Source: three-view drawing plus pictorial views. Frame: mm from the lowest corner of the part. A direction names the side the tool comes from. Round coordinates to 2 decimals unless told otherwise and drop trailing zeros. Loops run counter-clockwise (first coordinate to the right, second up) from the corner with the lowest first, then second, coordinate; pieces in that order, holes last. Notation, with made-up numbers: (58.25, 80.25) -> (96.25, 80.25) arc R19 ccw to (96.25, 90.25) -> close; hole circle Ø10 at (70, 81.5). An arc over 180 degrees is marked (long way). Put each result on its own line as item: value. Start each with the question number.
1. Cut plane C-C (z = 115.5). Return the cut outline in (x, y), then the cut area to 3 significant figures.
2. Material intervals for L1, parallel to X at y = 25.5, z = 113; L2, parallel to Y at x = 23, z = 108; L3, parallel to Z at x = 92, y = 56, sorted ascending.
3. Cut plane A-A (y = 26.5). State how many separate pieces and enclosed holes the cut face has, then the cut area to 3 significant figures.
4. Set-up query: the marked faces 1, 2, 3, 4 and 5. Return all of +Z, -Z, +X, -X, +Y, -Y with unobstructed straight access to the full face (end or side cutting, diameter ignored); none if empty.
5. Cut plane D-D (y = 46). Return the cut outline in (x, z).
6. Cut plane B-B (x = 101). Return the cut outline in (y, z).
7. Contact query for flat-ended pins moving along their axis: pin 1 (1.5 mm diameter, centred on y = 18, z = 63, fed in from -X); pin 2 (19 mm diameter, centred on x = 98, y = 34, fed in from -Z); pin 3 (7 mm diameter, centred on x = 123, z = 79.5, fed in from -Y); pin 4 (5 mm diameter, centred on x = 53.5, y = 20, fed in from +Z). Output: stop coordinate, or through.
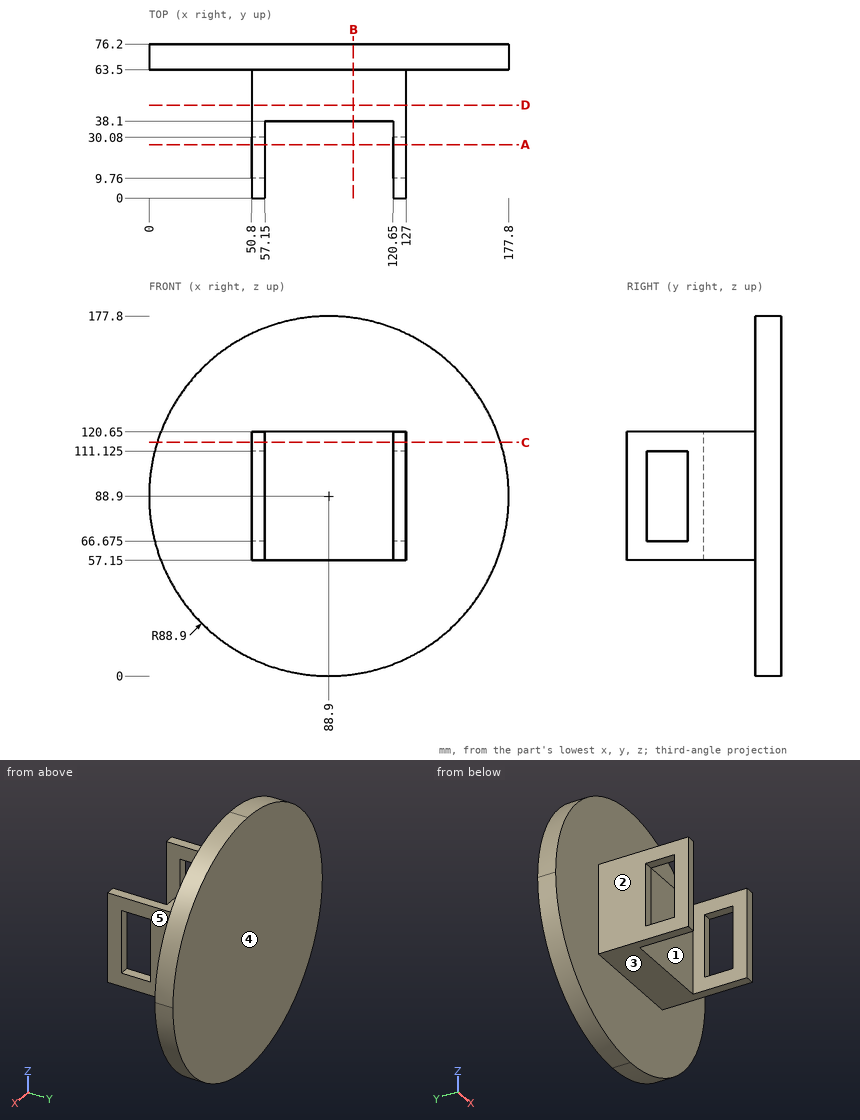
Solution:
1. outline: (4.07, 63.5) -> (50.8, 63.5) -> (50.8, 0) -> (57.15, 0) -> (57.15, 38.1) -> (120.65, 38.1) -> (120.65, 0) -> (127, 0) -> (127, 63.5) -> (173.73, 63.5) -> (173.73, 76.2) -> (4.07, 76.2) -> close
1. area: 4,570 mm^2
2. L1: x = 50.8 to 57.15, 120.65 to 127
2. L2: y = 63.5 to 76.2
2. L3: z = 57.15 to 120.65
3. separate pieces: 4
3. enclosed holes: 0
3. area: 242 mm^2
4. face 1: +Z, -Z, -Y
4. face 2: +Z, -Z, -X, -Y
4. face 3: -Z, +X, -X, -Y
4. face 4: +Z, -Z, +X, -X, +Y
4. face 5: +Z, -Z, +X, -Y
5. outline: (50.8, 57.15) -> (127, 57.15) -> (127, 120.65) -> (50.8, 120.65) -> close
6. outline: (38.1, 57.15) -> (63.5, 57.15) -> (63.5, 0.83) -> (76.2, 0.83) -> (76.2, 176.97) -> (63.5, 176.97) -> (63.5, 120.65) -> (38.1, 120.65) -> close
7. pin 1: stops at x = 50.8
7. pin 2: stops at z = 57.15
7. pin 3: stops at y = 0
7. pin 4: stops at z = 120.65
